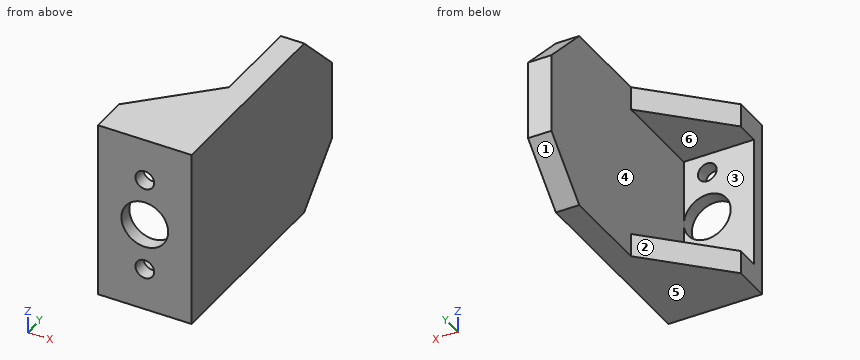
Autodesk Inventor part; units mm, degrees
ref_plane "YZ Plane" through (0, 0, 0) normal (1, 0, 0) x (0, 1, 0)
ref_plane "XZ Plane" through (0, 0, 0) normal (0, 1, 0) x (-1, 0, 0)
ref_plane "XY Plane" through (0, 0, 0) normal (0, 0, 1) x (1, 0, 0)
sketch "Эскиз1" plane through (0, 0, 0) normal (0, 1, 0) x (-1, 0, 0)
  line L0 (-10, 19) -> (10, 19)
  line L1 (10, 19) -> (10, -19)
  line L2 (10, -19) -> (-10, -19)
  line L3 (-10, -19) -> (-10, 19)
  line L4 (-10, 19) -> (10, -19) construction
  line L5 (10, 19) -> (-10, -19) construction
  circle A0 centre (0, 0) radius 5
  line L6 (0, 0) -> (0, 10)
  line L7 (0, 10) -> (0, -10)
  circle A1 centre (0, 10) radius 2
  circle A2 centre (0, -10) radius 2
  dimension "d0" = 20
  dimension "d1" = 38
  dimension "d2" = 10
  dimension "d3" = 10
  dimension "d4" = 20
  dimension "d5" = 4
  dimension "d6" = 4
extrude "Выдавливание1" add sketch "Эскиз1" along normal blind 3
sketch "Эскиз2" plane through (0, 3, 0) normal (0, 1, 0) x (1, 0, 0)
  line L0 (-10, -19) -> (10, -19)
  line L1 (10, -19) -> (5, -19)
  line L2 (5, -19) -> (5, 19)
  line L3 (5, 19) -> (10, 19)
  line L4 (10, 19) -> (10, -19)
  point P0 (0, 0)
  dimension "d9" = 38
  dimension "d10" = 5
extrude "Выдавливание2" add sketch "Эскиз2" along normal blind 50
chamfer "Фаска1" distance 10.5 angle 45 2 edges at (7.5, 53, -19) (7.5, 53, 19)
sketch "Эскиз3" plane through (0, 3, 0) normal (0, 1, 0) x (1, 0, 0)
  line L0 (-10, 19) -> (10, 19)
  line L1 (5, 0) -> (5, 19)
  line L2 (-10, 19) -> (5, 19)
  line L3 (5, 19) -> (5, 14)
  line L4 (5, 14) -> (-10, 14)
  line L5 (-10, 14) -> (-10, 19)
  line L6 (10, -19) -> (-10, -19)
  line L7 (5, -8.5) -> (5, -19)
  line L8 (-10, -19) -> (5, -19)
  line L9 (5, -19) -> (5, -14)
  line L10 (5, -14) -> (-10, -14)
  line L11 (-10, -14) -> (-10, -19)
  point P0 (0, 0)
  dimension "d16" = 5
  dimension "d17" = 5
extrude "Выдавливание3" add sketch "Эскиз3" along normal blind 20
chamfer "Фаска2" distance 15 angle 45 2 edges at (-10, 23, -16.5) (-10, 23, 16.5)
properties part number "МД.001.1005 - Прихват"
Build history of the part. All positions in model axes, mm. Face numbers are marked on the shaded views. A direction names the side the tool comes from. Round coordinates to 2 decimals unless told otherwise and drop trailing zeros. Loops run counter-clockwise (first coordinate to the right, second up) from the corner with the lowest first, then second, coordinate; pieces in that order, holes last. Notation, with made-up numbers: M 81,12.25 L 102,12.25 A21 cw 102,37.25 Z; hole C 59.25,0 d9. An arc over 180 degrees is marked long. Answer as CSV lines item,"result".
1. 3-axis set-ups, long thin cutter, end or side, ignore diameter. For the marked faces 5 and 6: which of +Z, -Z, +X, -X, +Y, -Y reach the whole face in a straight line?
Resolved:
face 5,"-Z, +X, -X, +Y, -Y"
face 6,"-X, +Y"
2. Cut at D-D on x = 0. Write the cut outline in (y, z), then the cut area to 3 significant figures.
Resolved:
outline,"M 0,-19 L 18,-19 L 18,-14 L 3,-14 L 3,-12 L 0,-12 Z; M 0,-8 L 3,-8 L 3,-5 L 0,-5 Z; M 0,5 L 3,5 L 3,8 L 0,8 Z; M 0,12 L 3,12 L 3,14 L 18,14 L 18,19 L 0,19 Z"
area,"210 mm²"
3. Cut at A-A on z = 10. Write the cut outline in (x, y).
Resolved:
outline,"M -10,0 L -2,0 L -2,3 L -10,3 Z; M 2,0 L 10,0 L 10,51.5 L 5,51.5 L 5,3 L 2,3 Z"
4. Cut at C-C on y = 4.5. Write the cut outline in (x, z), then the cut area to 3 significant figures.
Resolved:
outline,"M -10,-19 L 10,-19 L 10,19 L -10,19 L -10,14 L 5,14 L 5,-14 L -10,-14 Z"
area,"340 mm²"
5. Cut at B-B on x = 3.5. Write the cut outline in (y, z), then the cut area to 3 significant figures.
Resolved:
outline,"M 0,-19 L 21.5,-19 L 21.5,-14 L 3,-14 L 3,-3.57 L 0,-3.57 Z; M 0,3.57 L 3,3.57 L 3,14 L 21.5,14 L 21.5,19 L 0,19 Z"
area,"278 mm²"
6. Wall check: probe 1 along Z at (x, y) = (0, 1.5); probe 2 along X at (y, z) = (1, -10); probe 3 along Z at (x, y) = (1, 10). Give the ranges that are in metal, low to high. Write a range as [from, to].
Resolved:
probe 1,"z = [-19, -12], [-8, -5], [5, 8], [12, 19]"
probe 2,"x = [-10, -2], [2, 10]"
probe 3,"z = [-19, -14], [14, 19]"
7. Two-plate mould, pull along Z, no slides. Class the marked faces 1, 2, 3 and 4: released by +Z, released by -Z, zero draft, split by the parting line, or undercut.
Resolved:
face 1,"released by -Z"
face 2,"zero draft"
face 3,"undercut"
face 4,"undercut"
